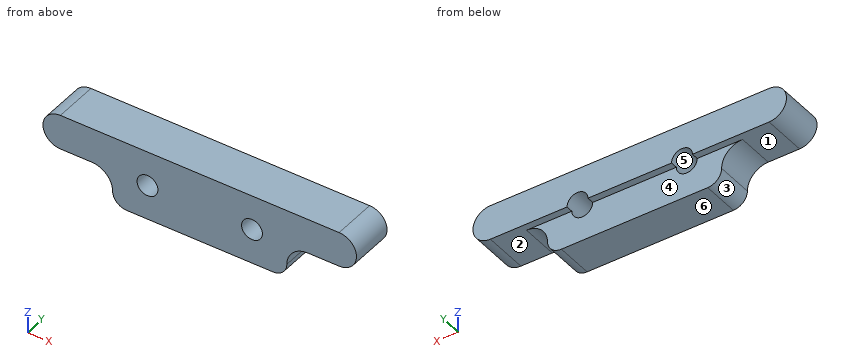
from build123d import *

# Parameters (mm, degrees)
BOSS_EXTRUDE1_DEPTH         = 6.35
TAP_DRILL_FOR_M4X0_7_TAP1_D = 3
FILLET1_R                   = 3
CUT_EXTRUDE1_START          = -7.5
CUT_EXTRUDE1_OUTLINE_W      = 34
CUT_EXTRUDE1_OUTLINE_H      = 1
CUT_EXTRUDE1_DEPTH          = 5


# Read off the part's stored shape, not the designer's step: Cut-Extrude1
with BuildPart() as part:
    # Sketch1 → Boss-Extrude1 (new body)
    with BuildSketch(Plane(origin=(0, 0, 0), x_dir=(1, 0, 0), z_dir=(0, 1, 0))):
        with BuildLine():
            Line((-20, -2.5), (20, -2.5))
            ThreePointArc((20, -2.5), (22.5, 0), (20, 2.5))
            Line((20, 2.5), (-20, 2.5))
            ThreePointArc((-20, 2.5), (-22.5, 0), (-20, -2.5))
        make_face()
        with BuildLine():
            Line((-12.5, 5.5), (-12.5, 2.5))
            Line((-12.5, 2.5), (12.5, 2.5))
            Line((12.5, 2.5), (12.5, 5.5))
            ThreePointArc((12.5, 5.5), (11.914213562, 6.914213562), (10.5, 7.5))
            Line((10.5, 7.5), (-10.5, 7.5))
            ThreePointArc((-10.5, 7.5), (-11.914213562, 6.914213562), (-12.5, 5.5))
        make_face()
    extrude(amount=BOSS_EXTRUDE1_DEPTH)

    # Tap Drill for M4x0.7 Tap1 (through all)
    with Locations(Plane(origin=(0, 6.35, 0), x_dir=(1, 0, 0), z_dir=(0, 1, 0))):
        with Locations((-7.5, 2.5), (7.5, 2.5)):
            Hole(TAP_DRILL_FOR_M4X0_7_TAP1_D / 2)

    # Fillet1
    fillet1_edges = [part.edges().sort_by_distance(p)[0] for p in [
        (12.5, 3.175, -2.5),
        (-12.5, 3.175, -2.5),
    ]]
    fillet(fillet1_edges, radius=FILLET1_R - 0.0001)  # a hair under: the kernel refuses the full size

    # Cut-Extrude1 outline → Cut-Extrude1 (cut)
    with BuildSketch(Plane.XY.offset(CUT_EXTRUDE1_START)):
        with Locations((0, 5.85)):
            Rectangle(CUT_EXTRUDE1_OUTLINE_W, CUT_EXTRUDE1_OUTLINE_H)
    extrude(amount=CUT_EXTRUDE1_DEPTH, mode=Mode.SUBTRACT)


solid = part.part
Read the model definition and answer for the solid it produces. Units are mm, in the model's axes. Face numbers are marked on the shaded views. A direction names the side the tool comes from. Round coordinates to 2 decimals unless told otherwise and drop trailing zeros. Order: outer loops, then holes, each group sorted by start corner. A loop starts at its lowest first (then second) coordinate and runs counter-clockwise, first axis right, second up. Notation, with made-up numbers: (-23, 79) - (-12, 79) arc R28 cw to (-12, 118) - close; hole circle Ø4 at (64.25, -16.75). An arc over 180 degrees is marked (long way). Use one line per item in the form item = value. Start each with the question number.
(1) The part is cut by section A-A (x = 7.5). Give the vertices of the cut face in (y, z), then the cut area to 4 significant figures.
(2) Flat-ended cylindrical pins translate along their axes: pin 1 Ø1.5 at (x, z) = (0.5, -6) entering from +Y; pin 2 Ø3 at (y, z) = (5, -2.5) entering from +X. Find the tip coordinate at first contact, or state that the pin passes through.
(3) Find the intervals of material crossed by line 1 along Z through (x, y) = (-7.5, 4.5); line 2 along X through (y, z) = (4.5, -3); line 3 along Z through (x, y) = (-16.5, 3.5), in increasing order. Write a range as from..to.
(4) The part is cut by section C-C (y = 4.5). Count the separate pieces of the cut face and the enclosed holes in it, then the cut area to 3 significant figures.
(5) The part is cut by section B-B (z = -1.5). Give the vertices of the cut face in (x, y), then the cut area to 3 significant figures.
(6) Determine the mould class of the marked faces 4, 5 and 6 for opening direction Z: +Z half, -Z half, draft (parallel to the pull), parting line (faces both ways), or undercut.
(7) For the marked faces 1, 2 and 3, determine the directions among +Z, -Z, +X, -X, +Y, -Y from which every point of the face is accessible in a straight line to the end or side of a thin tool.
(8) The part is cut by section D-D (x = -1.5). Give the vertices of the cut face in (y, z).
Checked values:
q1.outline = (0, -7.5) - (5.35, -7.5) - (5.35, -4) - (0, -4) - close; (0, -1) - (6.35, -1) - (6.35, 2.5) - (0, 2.5) - close
q1.area = 40.95 mm^2
q2.pin_1 = 5.35
q2.pin_2 = 22.29
q3.line_1 = -7.5..-4, -1..2.5
q3.line_2 = -13.84..-8.91, -6.09..6.09, 8.91..13.84
q3.line_3 = -2.5..2.5
q4.separate_pieces = 1
q4.enclosed_holes = 2
q4.area = 333 mm^2
q5.outline = (-22, 0) - (-8.62, 0) - (-8.62, 6.35) - (-22, 6.35) - close; (-6.38, 0) - (6.38, 0) - (6.38, 6.35) - (-6.38, 6.35) - close; (8.62, 0) - (22, 0) - (22, 6.35) - (8.62, 6.35) - close
q5.area = 251 mm^2
q6.face_4 = draft
q6.face_5 = undercut
q6.face_6 = -Z half
q7.face_1 = -Z, -X, +Y
q7.face_2 = -Z, +X, +Y
q7.face_3 = -Z, -X, +Y, -Y
q8.outline = (0, -7.5) - (5.35, -7.5) - (5.35, -2.5) - (6.35, -2.5) - (6.35, 2.5) - (0, 2.5) - close
